Check sheet for the modelled part. Datum: model origin and axes. Units: mm. Coordinates: 2 decimals unless noted, no trailing zeros. Write each loop counter-clockwise with the first axis right and the second up, starting at its lowest first coordinate (ties: lowest second). Pieces come first, ordered by that corner, then holes. Notation, with made-up numbers: M -27.5,29 L 31.5,29 A24 cw 31.5,46 Z; hole C 76,75 d3. An arc over 180 degrees is marked long. Answer as CSV lines item,"result". Start each with the question number.
Q1. Sectioned sample at C-C, the plane y = 31. Record the cut outline in (x, z).
Q2. Thickness scan on line 1 along Y through (x, z) = (-23.57, 1.85); line 2 along Y through (x, z) = (-1, 0.4); line 3 along X through (y, z) = (-7.5, 2.05). Record the ranges inside material, lowest first. Write a range as from..to.
Q3. Sectioned sample at B-B, the plane z = 0.8. Record the cut outline in (x, y), then the cut area to 3 significant figures.
Q4. Depth check by flat-ended pin: pin 1 Ø2 at (x, z) = (193, 1.5) entering from +Y; pin 2 Ø4 at (x, y) = (88.5, -14.5) entering from -Z; pin 3 Ø4.5 at (x, y) = (23.57, -23.57) entering from +Z. Enter the tip coordinate at first touch or a pass-through.
Q5. Sectioned sample at D-D, the plane x = 165. Record the cut outline in (y, z), then the cut area to 3 significant figures.
Q6. Sectioned sample at A-A, the plane y = 0. Record the cut outline in (x, z).
from build123d import *

# Parameters (mm, degrees)
SKETCH_1_R      = 2.5
SKETCH_1_R_2    = 9.5
EXTRUDE_1_DEPTH = 4


with BuildPart() as part:
    # 草图1 → 凸台-拉伸1 (new body)
    with BuildSketch(Plane.XY):
        with BuildLine():
            Line((31.224989992, 25), (311.341198994, 25))
            ThreePointArc((311.341198994, 25), (382.566188986, 0), (311.341198994, -25))
            Line((311.341198994, -25), (31.224989992, -25))
            ThreePointArc((31.224989992, -25), (-40, 0), (31.224989992, 25))
        make_face()
        with Locations((-23.57, 23.57)):
            Circle(SKETCH_1_R, mode=Mode.SUBTRACT)
        with Locations((23.57, 23.57)):
            Circle(SKETCH_1_R, mode=Mode.SUBTRACT)
        with Locations((23.57, -23.57)):
            Circle(SKETCH_1_R, mode=Mode.SUBTRACT)
        with Locations((-23.57, -23.57)):
            Circle(SKETCH_1_R, mode=Mode.SUBTRACT)
        with Locations((342.566188986, 0)):
            Circle(SKETCH_1_R_2, mode=Mode.SUBTRACT)
        Circle(SKETCH_1_R_2, mode=Mode.SUBTRACT)
    extrude(amount=EXTRUDE_1_DEPTH)


solid = part.part
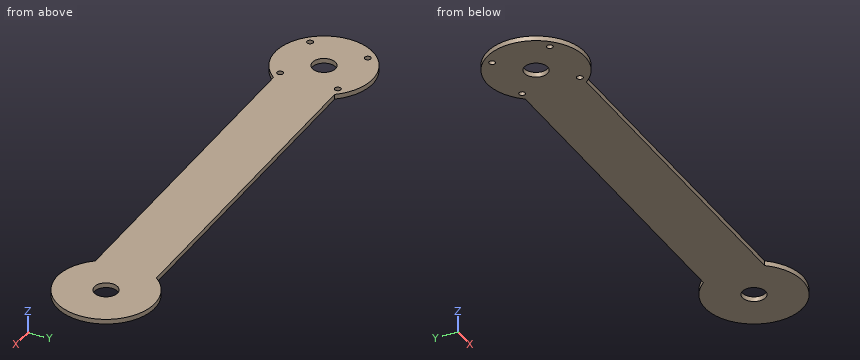
Output:
1,outline,"M -25.28,0 L 25.28,0 L 25.28,4 L -25.28,4 Z; M 317.29,0 L 367.84,0 L 367.84,4 L 317.29,4 Z"
2,line 1,"y = -32.32..-26.07, -21.07..21.07, 26.07..32.32"
2,line 2,"y = -39.99..-9.45, 9.45..39.99"
2,line 3,"x = -39.29..-5.83, 5.83..336.74, 348.4..381.86"
3,outline,"M 31.22,-25 L 311.34,-25 A40 ccw long 311.34,25 L 31.22,25 A40 ccw long Z; hole C -23.57,-23.57 d5; hole C -23.57,23.57 d5; hole C 0,0 d19; hole C 23.57,-23.57 d5; hole C 23.57,23.57 d5; hole C 342.57,0 d19"
3,area,"22,800 mm^2"
4,pin 1,"stops at y = 25"
4,pin 2,"stops at z = 0"
4,pin 3,"passes through"
5,outline,"M -25,0 L 25,0 L 25,4 L -25,4 Z"
5,area,"200 mm^2"
6,outline,"M -40,0 L -9.5,0 L -9.5,4 L -40,4 Z; M 9.5,0 L 333.07,0 L 333.07,4 L 9.5,4 Z; M 352.07,0 L 382.57,0 L 382.57,4 L 352.07,4 Z"
